```python
from build123d import *

# Parameters (mm, degrees)
F2_R = 0.99999
F3_R = 1


# Not quite as in the source:
# - a fillet or chamfer is up to 0.001 mm smaller than in the source, because OpenCascade refuses the exact size


with BuildPart() as f1:
    # F0 (on Top) → F1 (revolve)
    with BuildSketch(Plane.XY):
        Polygon((-31.8053636701, 0), (0, 0), (0, 2), (-30, 2), (-38, 80), (-43, 80), (-43, 78), (-39.8053636701, 78), align=None)
    revolve(axis=Axis((0, 3.6410242221, 0), (0, -1, 0)))

    # F2 (radius 1 in the source; OpenCascade refuses exactly that, so slightly less here)
    f2_edges = [f1.edges().sort_by_distance(p)[0] for p in [
        (43, 80, 0),
        (43, 78, 0),
        (-43, 79, 0),
    ]]
    fillet(f2_edges, radius=F2_R)

    # F3
    f3_edges = [f1.edges().sort_by_distance(p)[0] for p in [
        (38, 80, 0),
    ]]
    fillet(f3_edges, radius=F3_R)


solid = f1.part
```
Work out the finished part from the listing and answer in its coordinate system (mm). A direction names the side the tool comes from. Coordinates: 2 decimals unless noted, no trailing zeros. Order: outer loops, then holes, each group sorted by start corner. A loop starts at its lowest first (then second) coordinate and runs counter-clockwise, first axis right, second up. Notation, with made-up numbers: M 41.25,-3 L 57.25,-3 A27 ccw 57.25,24 Z; hole C 83.25,-26.75 d5. An arc over 180 degrees is marked long. Use CSV: the item, a comma, the result in double quotes.
1) For faces 4 (the face through (-37.1, 78, 15.4)), 5 (the face through (7.37, 41.09, 33.2)), determine the directions among +Z, -Z, +X, -X, +Y, -Y from which every point of the face is accessible in a straight line to the end or side of a thin tool.
Worked out:
face 4,"-Y"
face 5,"+Y"
2) Section D-D on y = 53 is taken. Write down the section's boundary in (x, z), plus the area to 3 significant figures.
Worked out:
outline,"C 0,0 d74.48; hole C 0,0 d70.46"
area,"458 mm^2"
3) Section C-C on y = 26 is taken. Write down the section's boundary in (x, z), plus the area to 3 significant figures.
Worked out:
outline,"C 0,0 d68.94; hole C 0,0 d64.92"
area,"423 mm^2"
4) Consider line 1 (Y direction, x = -26.5, z = 10.5); line 2 (X direction, y = 16.5, z = -24); line 3 (Z direction, x = -18.5, y = 24.5). Determine where each line is inside the solid, lowest interval first. Write a range as [from, to].
Worked out:
line 1,"y = [0, 2]"
line 2,"x = [-23.37, -20.38], [20.38, 23.37]"
line 3,"z = [-28.9, -26.49], [26.49, 28.9]"
5) Flat-ended cylindrical pins translate along their axes: pin 1 Ø1.5 at (x, y) = (20.5, 19) entering from -Z; pin 2 Ø3 at (x, y) = (28.5, 69) entering from +Z; pin 3 Ø10 at (y, z) = (9, -30) entering from -X. Find the tip coordinate at first contact, or state that the pin passes through.
Worked out:
pin 1,"stops at z = -27.38"
pin 2,"stops at z = 27.99"
pin 3,"stops at x = -21.18"
6) Determine the mould class of faces 1 (the face through (0, 2, 0)), 2 (the face through (4.654, 38.454, -35.445)), 3 (the face through (12.2, 80, 37.1)) for opening direction Z: released by +Z, released by -Z, zero draft, split by the parting line, or undercut.
Worked out:
face 1,"undercut"
face 2,"split by the parting line"
face 3,"zero draft"
